Source: CAD feature listing. Evaluate the final solid. Frame: model axes, mm. A direction names the side the tool comes from. Give positions to 0.01 mm unless a question says otherwise; leave off trailing zeros. Loops run counter-clockwise (first coordinate to the right, second up) from the corner with the lowest first, then second, coordinate; pieces in that order, holes last. Notation, with made-up numbers: (32.25, -38) -> (41.25, -38) arc R10 cw to (41.25, -27) -> close; hole circle Ø3 at (30.5, -1). An arc over 180 degrees is marked (long way). Answer as a JSON object with one key per item and string values. Group by question number.
from build123d import *

# Parameters (mm, degrees)
SKETCH1_W           = 144
SKETCH1_H           = 51
BOSS_EXTRUDE1_DEPTH = 3
BOSS_EXTRUDE2_START = -3
SKETCH2_W           = 144
SKETCH2_H           = 51
SKETCH2_W_2         = 139
SKETCH2_H_2         = 46
BOSS_EXTRUDE2_DEPTH = 16
BOSS_EXTRUDE3_DEPTH = 16.5
SKETCH4_R           = 2
SKETCH4_R_2         = 1.5
CUT_EXTRUDE1_DEPTH  = 84.009035653
SKETCH5_R           = 0.762
CUT_EXTRUDE2_DEPTH  = 95.027921385


with BuildPart() as part:
    # Sketch1 → Boss-Extrude1 (new body)
    with BuildSketch(Plane(origin=(0, 0, 0), x_dir=(1, 0, 0), z_dir=(0, 1, 0))):
        Rectangle(SKETCH1_W, SKETCH1_H)
    extrude(amount=BOSS_EXTRUDE1_DEPTH)

    # Sketch2 → Boss-Extrude2 (add)
    with BuildSketch(Plane(origin=(0, 3, 0), x_dir=(1, 0, 0), z_dir=(0, 1, 0)).offset(BOSS_EXTRUDE2_START)):
        Rectangle(SKETCH2_W, SKETCH2_H)
        Rectangle(SKETCH2_W_2, SKETCH2_H_2, mode=Mode.SUBTRACT)
    extrude(amount=BOSS_EXTRUDE2_DEPTH)

    # Sketch3 → Boss-Extrude3 (add)
    with BuildSketch(Plane(origin=(0, 16, 0), x_dir=(1, 0, 0), z_dir=(0, 1, 0))):
        Polygon((-72, 25.5), (-72, 12.5), (-69.5, 12.5), (-69.5, 23), (-47, 23), (-47, 25.5), align=None)
        Polygon((47, 25.5), (72, 25.5), (72, 12.5), (69.5, 12.5), (69.5, 23), (47, 23), align=None)
        Polygon((72, -25.5), (72, -12.5), (69.5, -12.5), (69.5, -23), (47, -23), (47, -25.5), align=None)
        Polygon((-47, -25.5), (-72, -25.5), (-72, -12.5), (-69.5, -12.5), (-69.5, -23), (-47, -23), align=None)
    extrude(amount=BOSS_EXTRUDE3_DEPTH)

    # Sketch4 → Cut-Extrude1 (cut, through all)
    with BuildSketch(Plane.XZ):
        with Locations(Location((-45, -13, 0), (0, 0, 270))):
            Circle(SKETCH4_R)
        with Locations(Location((-45, 13, 0), (0, 0, 270))):
            Circle(SKETCH4_R)
        with Locations(Location((45, 13, 0), (0, 0, 270))):
            Circle(SKETCH4_R)
        with Locations(Location((45, -13, 0), (0, 0, 270))):
            Circle(SKETCH4_R)
        with Locations(Location((-50, -0.45, 0), (0, 0, 270))):
            Circle(SKETCH4_R_2)
        with Locations(Location((50, -0.45, 0), (0, 0, 270))):
            Circle(SKETCH4_R_2)
    extrude(amount=-CUT_EXTRUDE1_DEPTH, mode=Mode.SUBTRACT)

    # Sketch5 → Cut-Extrude2 (cut, through all)
    with BuildSketch(Plane.XY.offset(25.5)):
        with Locations((-55.88, 8)):
            Circle(SKETCH5_R)
        with Locations((55.88, 8)):
            Circle(SKETCH5_R)
        with Locations((0, 8)):
            Circle(SKETCH5_R)
    extrude(amount=-CUT_EXTRUDE2_DEPTH, mode=Mode.SUBTRACT)


solid = part.part
(1) Section query A-A on x = -50. Return the cut outline in (y, z), plus the area to 4 significant figures.
(2) Material intervals for line 1 (X direction, y = 3.5, z = -4.5); line 2 (Z direction, x = 2, y = 11); line 3 (Y direction, x = -55.88, z = -24.15), sorted ascending. Write a range as from..to.
(3) First-contact query: pin 1 (0.8 mm diameter, centred on x = 71, z = -2, fed in from +Y); pin 2 (8 mm diameter, centred on x = 31.5, z = 1, fed in from +Y). Flat tips, straight axial feed; report the tip coordinate or a pass-through.
(4) Section query D-D on y = 10.5. Return the cut outline in (x, z).
(5) Section query B-B on y = 19. Return the cut outline in (x, z), plus the area to 3 significant figures.
(6) Access query for faces 4 (the face through (-1, 16, 24)), 5 (the face through (48.536, 1.479, -0.125)), 6 (the face through (-1, 3, 0)), 7 (the face through (71, 16, 0)). Directions: +Z, -Z, +X, -X, +Y, -Y. A direction counts if a zero-diameter tool reaches every point of the face in a straight line with its end or side. Return the directions, or none.
(7) Mould query, pull axis Z, two halves, no side actions, for faces 1 (the face through (1, 12, -25.5)), 2 (the face through (-51.464, 1.479, -0.125)), 3 (the face through (72, 12, 0)). Classes: pulls with the +Z half, pulls with the -Z half, needs draft (parallel to the pull), parting line crosses it, or undercut.
(8) Section query C-C on z = -20. Return the cut outline in (x, y).
Result:
{
 "1": {"outline": "(0, -25.5) -> (32.5, -25.5) -> (32.5, -23) -> (3, -23) -> (3, -1.95) -> (0, -1.95) -> close; (0, 1.05) -> (3, 1.05) -> (3, 23) -> (32.5, 23) -> (32.5, 25.5) -> (0, 25.5) -> close", "area": "291.5 mm²"},
 "2": {"line 1": "-72..-69.5, 69.5..72", "line 2": "-25.5..-23, 23..25.5", "line 3": "0..7.24, 8.76..32.5"},
 "3": {"pin 1": "y = 16", "pin 2": "y = 3"},
 "4": {"outline": "(-72, -25.5) -> (72, -25.5) -> (72, 25.5) -> (-72, 25.5) -> close; hole (-69.5, -23) -> (69.5, -23) -> (69.5, 23) -> (-69.5, 23) -> close"},
 "5": {"outline": "(-72, -25.5) -> (-47, -25.5) -> (-47, -23) -> (-69.5, -23) -> (-69.5, -12.5) -> (-72, -12.5) -> close; (-72, 12.5) -> (-69.5, 12.5) -> (-69.5, 23) -> (-47, 23) -> (-47, 25.5) -> (-72, 25.5) -> close; (47, -25.5) -> (72, -25.5) -> (72, -12.5) -> (69.5, -12.5) -> (69.5, -23) -> (47, -23) -> close; (47, 23) -> (69.5, 23) -> (69.5, 12.5) -> (72, 12.5) -> (72, 25.5) -> (47, 25.5) -> close", "area": "355 mm²"},
 "6": {"face 4": "+Z, -Z, +Y", "face 5": "+Y, -Y", "face 6": "+Y", "face 7": "+X, -X, +Y"},
 "7": {"face 1": "pulls with the -Z half", "face 2": "undercut", "face 3": "needs draft"},
 "8": {"outline": "(-72, 0) -> (72, 0) -> (72, 32.5) -> (69.5, 32.5) -> (69.5, 3) -> (-69.5, 3) -> (-69.5, 32.5) -> (-72, 32.5) -> close"}
}
